```python
from build123d import *

# Parameters (mm, degrees)
SKETCH1_W           = 110
SKETCH1_H           = 110
BOSS_EXTRUDE1_DEPTH = 3
BOSS_EXTRUDE2_START = -2
BOSS_EXTRUDE2_DEPTH = 32
FILLET2_R           = 1


with BuildPart() as part:
    # Sketch1 → Boss-Extrude1 (new body)
    with BuildSketch(Plane(origin=(0, 0, 0), x_dir=(1, 0, 0), z_dir=(0, 1, 0))):
        Rectangle(SKETCH1_W, SKETCH1_H)
    extrude(amount=BOSS_EXTRUDE1_DEPTH)

    # Sketch2 → Boss-Extrude2 (add)
    with BuildSketch(Plane.XZ.offset(BOSS_EXTRUDE2_START)):
        Polygon((-39.393398282, 44.393398282), (-41.893398282, 48.723525301), (-46.893398282, 48.723525301), (-49.393398282, 44.393398282), (-46.893398282, 40.063271263), (-41.893398282, 40.063271263), align=None)
        Polygon((41.893398282, 40.063271263), (39.393398282, 44.393398282), (41.893398282, 48.723525301), (46.893398282, 48.723525301), (49.393398282, 44.393398282), (46.893398282, 40.063271263), align=None)
        Polygon((39.393398282, -44.393398282), (41.893398282, -48.723525301), (46.893398282, -48.723525301), (49.393398282, -44.393398282), (46.893398282, -40.063271263), (41.893398282, -40.063271263), align=None)
        Polygon((-41.893398282, -40.063271263), (-39.393398282, -44.393398282), (-41.893398282, -48.723525301), (-46.893398282, -48.723525301), (-49.393398282, -44.393398282), (-46.893398282, -40.063271263), align=None)
    extrude(amount=BOSS_EXTRUDE2_DEPTH)

    # Fillet2
    fillet2_edges = [part.edges().sort_by_distance(p)[0] for p in [
        (55, 3, 0),
        (0, 3, -55),
        (-55, 3, 0),
        (0, 0, -55),
        (55, 0, 0),
        (0, 0, 55),
        (-55, 0, 0),
        (-55, 1.5, -55),
        (55, 1.5, -55),
        (55, 1.5, 55),
        (-55, 1.5, 55),
        (0, 3, 55),
    ]]
    fillet(fillet2_edges, radius=FILLET2_R)


solid = part.part
```
Build history of the part. All positions in model axes, mm. A direction names the side the tool comes from. Round coordinates to 2 decimals unless told otherwise and drop trailing zeros. Write each loop counter-clockwise with the first axis right and the second up, starting at its lowest first coordinate (ties: lowest second). Pieces come first, ordered by that corner, then holes. Notation, with made-up numbers: (51, -38) - (68, -38) arc R23 ccw to (68, -20) - close; hole circle Ø4 at (29, 47). An arc over 180 degrees is marked (long way). Answer as CSV lines item,"result".
Q1. Drill centre lines: probe 1 along Z at (x, y) = (43.5, -16); probe 2 along Z at (x, y) = (40.5, -13.5); probe 3 along Y at (x, z) = (26, -5). Where is each one in solid material? Low to high. Write a range as [from, to].
Report:
probe 1,"z = [-48.72, -40.06], [40.06, 48.72]"
probe 2,"z = [-46.31, -42.48], [42.48, 46.31]"
probe 3,"y = [0, 3]"
Q2. Tool access for faces 4 (the flat face through (44, -15, -48.724)), 5 (the flat face through (-44, -15, 40.063)), 6 (the flat face through (-40.626, -14.79, -46.528)): list every direction of +Z, -Z, +X, -X, +Y, -Y with a clear straight run to the whole face (end or side of a thin tool).
Report:
face 4,"-Z, +X, -X, -Y"
face 5,"+X, -X, -Y"
face 6,"-Z, -Y"
Q3. Drop flat-ended pins along their axis: pin 1 (2.5 mm diameter, centred on x = 45, y = -14, fed in from -Z); pin 2 (4 mm diameter, centred on x = 44.5, y = -18.5, fed in from +Z); pin 3 (12 mm diameter, centred on x = 27, z = 2.5, fed in from -Y). Give the stop position or say it passes through.
Report:
pin 1,"stops at z = -48.72"
pin 2,"stops at z = 48.72"
pin 3,"stops at y = 0"
Q4. Cut at A-A (y = -23.5). Write the cut outline in (x, z).
Report:
outline,"(-49.39, -44.39) - (-46.89, -48.72) - (-41.89, -48.72) - (-39.39, -44.39) - (-41.89, -40.06) - (-46.89, -40.06) - close; (-49.39, 44.39) - (-46.89, 40.06) - (-41.89, 40.06) - (-39.39, 44.39) - (-41.89, 48.72) - (-46.89, 48.72) - close; (39.39, -44.39) - (41.89, -48.72) - (46.89, -48.72) - (49.39, -44.39) - (46.89, -40.06) - (41.89, -40.06) - close; (39.39, 44.39) - (41.89, 40.06) - (46.89, 40.06) - (49.39, 44.39) - (46.89, 48.72) - (41.89, 48.72) - close"
Q5. Cut at D-D (x = -33). Write the cut outline in (y, z), and give its area (3 significant figures).
Report:
outline,"(0, -54) arc R1 ccw to (1, -55) - (2, -55) arc R1 ccw to (3, -54) - (3, 54) arc R1 ccw to (2, 55) - (1, 55) arc R1 ccw to (0, 54) - close"
area,"329 mm^2"
Q6. Pull direction X, two halves, no side cores. Call faces 1 (the flat face through (40.66, -14.79, -42.2)), 2 (the flat face through (44, -30, 44)), 3 (the flat face through (48.126, -14.79, 46.589)): +X half, -X half, draft (parallel to the pull), parting line (faces both ways), or undercut.
Report:
face 1,"undercut"
face 2,"draft"
face 3,"+X half"
Q7. Cut at C-C (z = 33.5). Write the cut outline in (x, y), and give its area (3 significant figures).
Report:
outline,"(-55, 1) arc R1 ccw to (-54, 0) - (54, 0) arc R1 ccw to (55, 1) - (55, 2) arc R1 ccw to (54, 3) - (-54, 3) arc R1 ccw to (-55, 2) - close"
area,"329 mm^2"
Q8. Cut at B-B (x = -45). Write the cut outline in (y, z), and give its area (3 significant figures).
Report:
outline,"(-30, -48.72) - (0, -48.72) - (0, -54) arc R1 ccw to (1, -55) - (2, -55) arc R1 ccw to (3, -54) - (3, 54) arc R1 ccw to (2, 55) - (1, 55) arc R1 ccw to (0, 54) - (0, 48.72) - (-30, 48.72) - (-30, 40.06) - (0, 40.06) - (0, -40.06) - (-30, -40.06) - close"
area,"849 mm^2"
